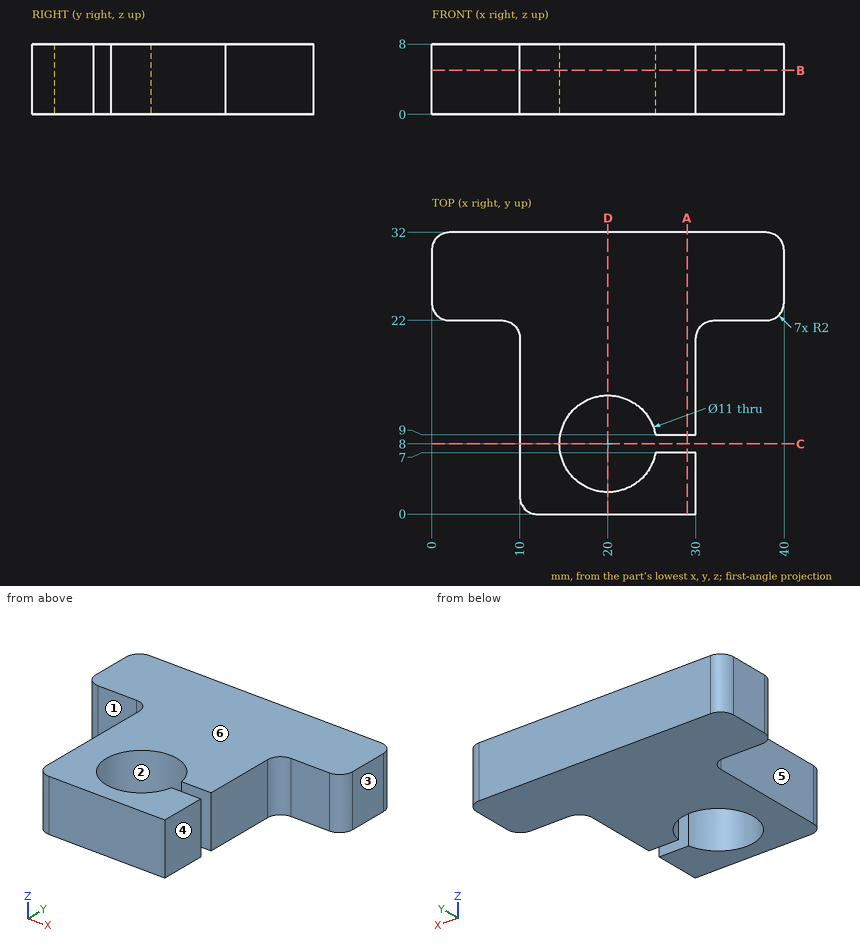
Could you check a few things on this drawing? It's one solid part, dimensions in mm from its lowest x, y, z. A direction names the side the tool comes from. Give positions to 0.01 mm unless a question says otherwise; leave off trailing zeros. Write each loop counter-clockwise with the first axis right and the second up, starting at its lowest first coordinate (ties: lowest second). Pieces come first, ordered by that corner, then holes. Notation, with made-up numbers: (51, -11.5) - (104, -11.5) arc R18 cw to (104, 15.5) - close; hole circle Ø9 at (49, -10). An arc over 180 degrees is marked (long way). Use CSV: the item, a comma, the result in double quotes. Start each with the question number.
Item 1: I want a section at C-C, the plane y = 8. Please give me the cut outline in (x, z), then the cut area to 3 significant figures.
Item 2: I want a section at A-A, the plane x = 29. Please give me the cut outline in (y, z).
Item 3: I'm going to push flat-ended pins straight in: pin 1 (4 mm diameter, centred on y = 16, z = 5, fed in from +X); pin 2 (4 mm diameter, centred on y = 21.5, z = 5.5, fed in from -X); pin 3 (3 mm diameter, centred on y = 9, z = 6.5, fed in from -X). Where does each tip first touch, or does it pass through?
Item 4: For the marked faces 4, 5 and 6, which set-ups out of +Z, -Z, +X, -X, +Y, -Y let a thin tool reach every point of the face, with its end or its side?
Item 5: I want a section at D-D, the plane x = 20. Please give me the cut outline in (y, z), then the cut area to 3 significant figures.
Item 6: I want a section at B-B, the plane z = 5. Please give me the cut outline in (x, y), then the cut area to 3 significant figures.
Item 7: If I drill on line 1 along Y through (x, z) = (20, 6.25); line 2 along X through (y, z) = (17.5, 2.75); line 3 along Y through (x, z) = (19, 4.5), over which ranges is the centre line in solid material (lowest first)?
Item 8: If we mould it in two halves opening along X, with no side actions, what happens to the marked faces 1, 2 and 3? For each: pulls with the +X half, pulls with the -X half, needs draft (parallel to the pull), parting line crosses it, or undercut.
Findings:
1,outline,"(10, 0) - (14.5, 0) - (14.5, 8) - (10, 8) - close"
1,area,"36.0 mm2"
2,outline,"(0, 0) - (7, 0) - (7, 8) - (0, 8) - close; (9, 0) - (32, 0) - (32, 8) - (9, 8) - close"
3,pin 1,"stops at x = 30"
3,pin 2,"stops at x = 0.06"
3,pin 3,"stops at x = 10"
4,face 4,"+Z, -Z, +X, -Y"
4,face 5,"+Z, -Z, -X, -Y"
4,face 6,"+Z, +X, -X, +Y, -Y"
5,outline,"(0, 0) - (2.5, 0) - (2.5, 8) - (0, 8) - close; (13.5, 0) - (32, 0) - (32, 8) - (13.5, 8) - close"
5,area,"168 mm2"
6,outline,"(0, 24) arc R2 ccw to (2, 22) - (8, 22) arc R2 cw to (10, 20) - (10, 2) arc R2 ccw to (12, 0) - (30, 0) - (30, 7) - (25.41, 7) arc R5.5 cw (long way) to (25.41, 9) - (30, 9) - (30, 20) arc R2 cw to (32, 22) - (38, 22) arc R2 ccw to (40, 24) - (40, 30) arc R2 ccw to (38, 32) - (2, 32) arc R2 ccw to (0, 30) - close"
6,area,"733 mm2"
7,line 1,"y = 0 to 2.5, 13.5 to 32"
7,line 2,"x = 10 to 30"
7,line 3,"y = 0 to 2.59, 13.41 to 32"
8,face 1,"needs draft"
8,face 2,"undercut"
8,face 3,"pulls with the +X half"
